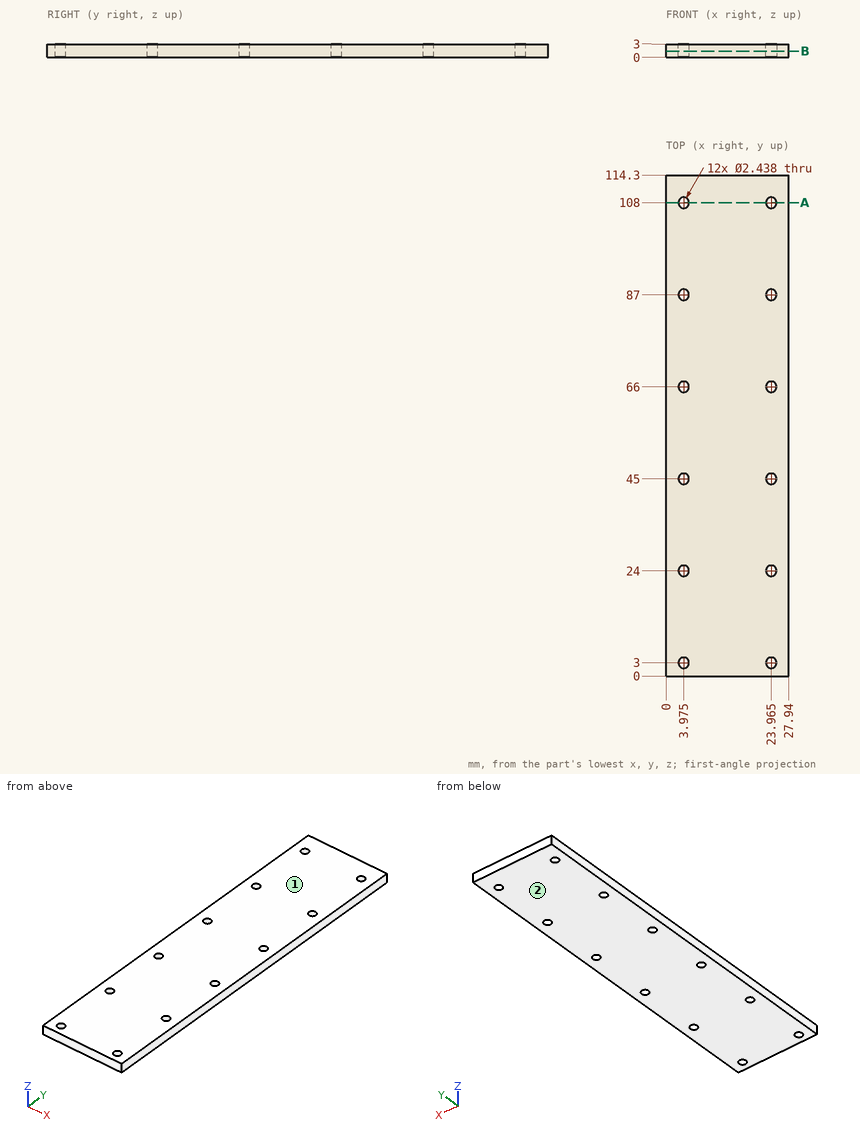
Geometry check sheet. Reference: drawing and pictorial views, mm from the part's lowest x, y, z. Round coordinates to 2 decimals unless told otherwise and drop trailing zeros. Order: outer loops, then holes, each group sorted by start corner. A loop starts at its lowest first (then second) coordinate and runs counter-clockwise, first axis right, second up. Notation, with made-up numbers: (36, 68) - (53, 68) arc R13 ccw to (53, 77) - close; hole circle Ø7 at (64, -4.75). An arc over 180 degrees is marked (long way). Use a Markdown table: item, result. Add a question column.
1) Section check A-A (y = 108). Record the cut outline in (x, z) (1 decimal).
2) Section check B-B (z = 1.4). Count the separate pieces of the cut face and the enclosed holes in it, then the cut area to 3 significant figures.
3) Thickness scan on line 1 along X through (y, z) = (66, 0.5) (1 decimal); line 2 along X through (y, z) = (86, 2.35) (1 decimal). Record the ranges inside material, lowest first.
4) Mould release check, pull along Z, two halves, no side actions. Record for the marked faces 1 and 2: released by +Z, released by -Z, zero draft, split by the parting line, or undercut.
Established:
| question | item | result |
|---|---|---|
| 1 | outline | (0, 0) - (2.8, 0) - (2.8, 3) - (0, 3) - close; (5.2, 0) - (22.7, 0) - (22.7, 3) - (5.2, 3) - close; (25.2, 0) - (27.9, 0) - (27.9, 3) - (25.2, 3) - close |
| 2 | separate pieces | 1 |
| 2 | enclosed holes | 12 |
| 2 | area | 3,140 mm2 |
| 3 | line 1 | 0 to 2.8, 5.2 to 22.7, 25.2 to 27.9 |
| 3 | line 2 | 0 to 3.3, 4.7 to 23.3, 24.7 to 27.9 |
| 4 | face 1 | released by +Z |
| 4 | face 2 | released by -Z |
